The listing builds one solid part. Answer for the finished solid, in the listing's coordinates (mm). Give positions to 0.01 mm unless a question says otherwise; leave off trailing zeros. Write each loop counter-clockwise with the first axis right and the second up, starting at its lowest first coordinate (ties: lowest second). Pieces come first, ordered by that corner, then holes. Notation, with made-up numbers: (-23.5, -25.75) -> (-18.5, -25.75) arc R14 cw to (-18.5, -2.75) -> close; hole circle Ø4 at (4.5, 69). An arc over 180 degrees is marked (long way). Put each result on its own line as item: value. Start each with the question number.
1) Find the intervals of material crossed by line 1 along Z through (x, y) = (2, 70.5); line 2 along Y through (x, z) = (2.6, 92.5); line 3 along Z through (x, y) = (1, 46), in increasing order. Write a range as from..to.
2) For a pull along Z with two mould halves and no side action, classify faces 1 (the flat face through (3.55, 29, 2)), 2 (the cylindrical face through (1.8, 108.5, -106.07)), 3 (the cylindrical face through (1.8, 108.57, 86)) as released by +Z, released by -Z, zero draft, split by the parting line, or undercut.
3) A cutting plane is placed at A-A (x = 1). Write down the section's boundary in (y, z), then the cut area to 3 significant figures.
4) A cutting plane is placed at B-B (y = 92). Write down the section's boundary in (x, z).
5) A flat-ended cylindrical pin translates along its axis: pin 1 Ø8 at (y, z) = (35.5, 81.5) entering from -X. Find the tip coordinate at first contact, or state that the pin passes through.
from build123d import *

# Parameters (mm, degrees)
F0_W     = 60
F0_H     = 195
F1_DEPTH = 3.55
F2_R     = 5


with BuildPart() as f1:
    # F0 (on Right) → F1 (new body)
    with BuildSketch(Plane.YZ):
        Polygon((50, 87.5), (50, 107.5), (-50, 107.5), (-50, -107.5), (50, -107.5), align=None)
        with Locations((80, -10)):
            Rectangle(F0_W, F0_H)
    extrude(amount=F1_DEPTH)

    # F2
    f2_edges = [f1.edges().sort_by_distance(p)[0] for p in [
        (1.775, 50, 87.5),
        (1.775, 50, 107.5),
        (1.775, 110, 87.5),
        (1.775, -50, 107.5),
        (1.775, 110, -107.5),
        (1.775, -50, -107.5),
    ]]
    fillet(f2_edges, radius=F2_R)


solid = f1.part
Reply:
1. line 1: z = -107.5..87.5
1. line 2: y = -50..50
1. line 3: z = -107.5..107.4
2. face 1: zero draft
2. face 2: released by -Z
2. face 3: released by +Z
3. outline: (-50, -102.5) arc R5 ccw to (-45, -107.5) -> (105, -107.5) arc R5 ccw to (110, -102.5) -> (110, 82.5) arc R5 ccw to (105, 87.5) -> (55, 87.5) arc R5 cw to (50, 92.5) -> (50, 102.5) arc R5 ccw to (45, 107.5) -> (-45, 107.5) arc R5 ccw to (-50, 102.5) -> close
3. area: 33,200 mm2
4. outline: (0, -107.5) -> (3.55, -107.5) -> (3.55, 87.5) -> (0, 87.5) -> close
5. pin 1: stops at x = 0
